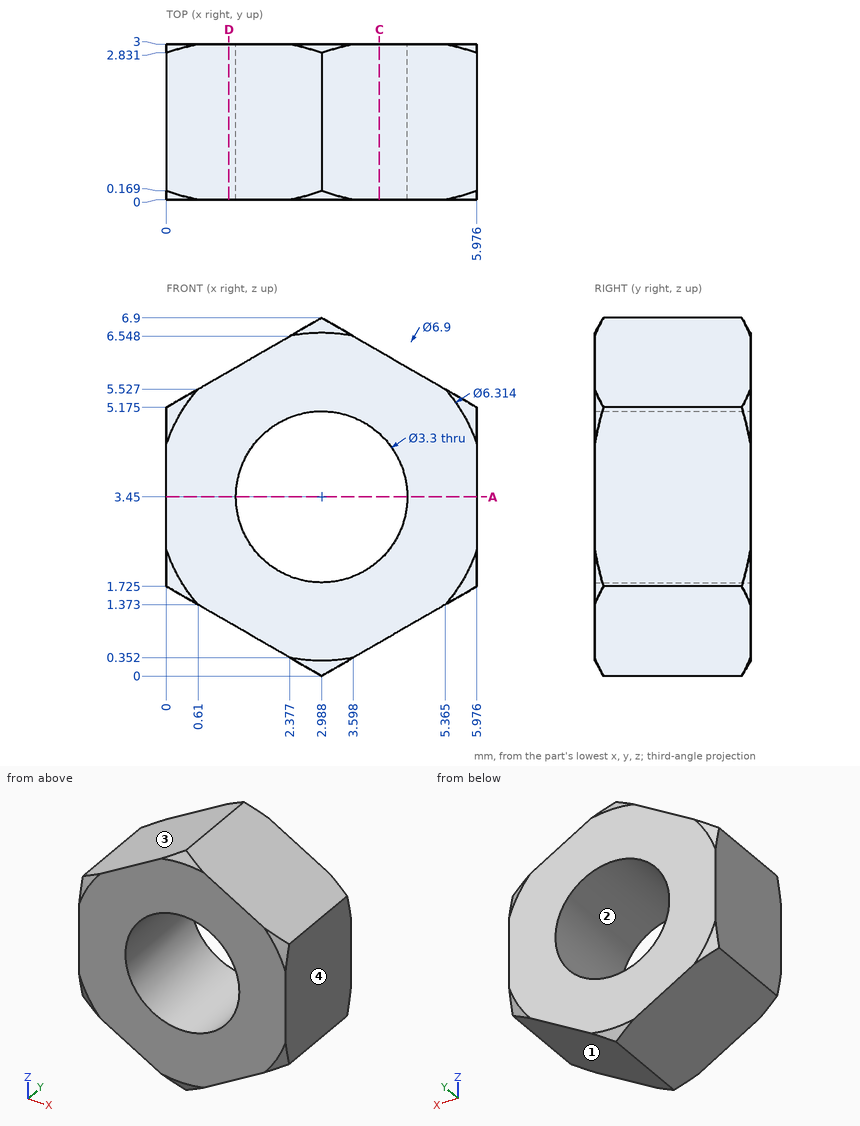
The figure shows three views and two pictorial views of one solid part (mm, origin at its lowest corner). Answer the questions. Coordinates: 2 decimals unless noted, no trailing zeros. Loops run counter-clockwise (first coordinate to the right, second up) from the corner with the lowest first, then second, coordinate; pieces in that order, holes last. Notation, with made-up numbers: (84.25, 85.25) -> (103.25, 85.25) arc R25 cw to (103.25, 102.25) -> close; hole circle Ø5 at (5.25, 50). An arc over 180 degrees is marked (long way). Write item = value, one per line. Start each with the question number.
1) The mould has two halves that part along Z. Classify the marked faces 1, 2, 3 and 4: released by +Z, released by -Z, zero draft, split by the parting line, or undercut.
2) A cutting plane is placed at A-A (z = 3.45). Give the vertices of the cut face in (x, y) (1 decimal).
3) A cutting plane is placed at D-D (x = 1.2). Give the vertices of the cut face in (y, z).
4) Straight lines are drawn through the part: line 1 (X direction, y = 1.6, z = 2.25) (1 decimal); line 2 (X direction, y = 1.6, z = 4.5) (1 decimal); line 3 (Z direction, x = 3.05, y = 1.15) (1 decimal). For each, find the intervals that lie inside material, in ascending order. Write a range as from..to.
5) A cutting plane is placed at C-C (x = 4.1). Give the vertices of the cut face in (y, z).
Responses:
q1.face_1 = released by -Z
q1.face_2 = undercut
q1.face_3 = released by +Z
q1.face_4 = zero draft
q2.outline = (0, 0) -> (1.3, 0) -> (1.3, 3) -> (0, 3) -> close; (4.6, 0) -> (6, 0) -> (6, 3) -> (4.6, 3) -> close
q3.outline = (0, 1.03) -> (3, 1.03) -> (3, 5.87) -> (0, 5.87) -> close
q4.line_1 = 0..1.9, 4.1..6
q4.line_2 = 0..1.7, 4.3..6
q4.line_3 = 0..1.8, 5.1..6.9
q5.outline = (0, 0.64) -> (3, 0.64) -> (3, 2.23) -> (0, 2.23) -> close; (0, 4.67) -> (3, 4.67) -> (3, 6.26) -> (0, 6.26) -> close
